from build123d import *

# Parameters (mm, degrees)
SKETCH2_R           = 2
BOSS_EXTRUDE1_DEPTH = 1.7
SKETCH3_W           = 98
SKETCH3_H           = 60
BOSS_EXTRUDE2_DEPTH = 3
SKETCH4_W           = 97
SKETCH4_H           = 40
BOSS_EXTRUDE3_DEPTH = 15
SKETCH5_W           = 6
SKETCH5_H           = 6
BOSS_EXTRUDE4_DEPTH = 3
SKETCH6_R           = 1.75
BOSS_EXTRUDE5_DEPTH = 0.65
SKETCH7_W           = 12.25
SKETCH7_H           = 11.75
BOSS_EXTRUDE6_DEPTH = 4.5
SKETCH8_R           = 6
BOSS_EXTRUDE7_DEPTH = 9.3
SKETCH9_W           = 45
SKETCH9_H           = 22.5
BOSS_EXTRUDE8_DEPTH = 10
SKETCH10_W          = 26.5
SKETCH10_H          = 26.5
BOSS_EXTRUDE9_DEPTH = 3.5
SKETCH11_W          = 76
SKETCH11_H          = 26
CUT_EXTRUDE1_DEPTH  = 0.5


with BuildPart() as part:
    # Sketch2 → Boss-Extrude1 (new body)
    with BuildSketch(Plane.XY):
        Polygon((75, 27.5), (75, -27.5), (-75, -27.5), (-75, 27.5), (-62.25, 27.5), (35.75, 27.5), align=None)
        with Locations((-72.5, -25)):
            Circle(SKETCH2_R, mode=Mode.SUBTRACT)
        with Locations((-72.5, 25)):
            Circle(SKETCH2_R, mode=Mode.SUBTRACT)
        with Locations((72.5, -25)):
            Circle(SKETCH2_R, mode=Mode.SUBTRACT)
        with Locations((72.5, 25)):
            Circle(SKETCH2_R, mode=Mode.SUBTRACT)
    extrude(amount=BOSS_EXTRUDE1_DEPTH)

    # Sketch3 → Boss-Extrude2 (add)
    with BuildSketch(Plane.XY):
        with Locations((-13.25, 6)):
            Rectangle(SKETCH3_W, SKETCH3_H)
    extrude(amount=-BOSS_EXTRUDE2_DEPTH)

    # Sketch4 → Boss-Extrude3 (add)
    with BuildSketch(Plane.XY):
        with Locations((-13.25, 5.5)):
            Rectangle(SKETCH4_W, SKETCH4_H)
    extrude(amount=-BOSS_EXTRUDE3_DEPTH)

    # Sketch5 → Boss-Extrude4 (add)
    with BuildSketch(Plane.XY):
        with Locations((62, 20)):
            Rectangle(SKETCH5_W, SKETCH5_H)
    extrude(amount=-BOSS_EXTRUDE4_DEPTH)

    # Sketch6 → Boss-Extrude5 (add)
    with BuildSketch(Plane(origin=(0, 0, -3), x_dir=(-1, 0, 0), z_dir=(0, 0, -1))):
        with Locations((-62, 20)):
            Circle(SKETCH6_R)
    extrude(amount=BOSS_EXTRUDE5_DEPTH)

    # Sketch7 → Boss-Extrude6 (add)
    with BuildSketch(Plane.XY):
        with Locations((62, 2.5)):
            Rectangle(SKETCH7_W, SKETCH7_H)
    extrude(amount=-BOSS_EXTRUDE6_DEPTH)

    # Sketch8 → Boss-Extrude7 (add)
    with BuildSketch(Plane.XY):
        with Locations((62, -17.5)):
            Circle(SKETCH8_R)
    extrude(amount=-BOSS_EXTRUDE7_DEPTH)

    # Sketch9 → Boss-Extrude8 (add)
    with BuildSketch(Plane.XY.offset(1.7)):
        with Locations((-6.5, 8.75)):
            Rectangle(SKETCH9_W, SKETCH9_H)
    extrude(amount=BOSS_EXTRUDE8_DEPTH)

    # Sketch10 → Boss-Extrude9 (add)
    with BuildSketch(Plane.XY.offset(1.7)):
        with Locations((-61.75, 6.25)):
            Rectangle(SKETCH10_W, SKETCH10_H)
    extrude(amount=BOSS_EXTRUDE9_DEPTH)

    # Sketch11 → Cut-Extrude1 (cut)
    with BuildSketch(Plane(origin=(0, 0, -15), x_dir=(-1, 0, 0), z_dir=(0, 0, -1))):
        with Locations((13.25, 5.5)):
            Rectangle(SKETCH11_W, SKETCH11_H)
    extrude(amount=-CUT_EXTRUDE1_DEPTH, mode=Mode.SUBTRACT)


solid = part.part
The listing builds one solid part. Answer for the finished solid, in the listing's coordinates (mm). A direction names the side the tool comes from. Round coordinates to 2 decimals unless told otherwise and drop trailing zeros. Write each loop counter-clockwise with the first axis right and the second up, starting at its lowest first coordinate (ties: lowest second). Pieces come first, ordered by that corner, then holes. Notation, with made-up numbers: (20.25, 84) - (48.25, 84) arc R22 cw to (48.25, 94) - close; hole circle Ø10 at (-17, -33.75). An arc over 180 degrees is marked (long way). Use a Markdown table: item, result. Add a question column.
1. The part is cut by section A-A (x = 29). Write down the section's boundary in (y, z), and give its area (4 significant figures).
2. Flat-ended cylindrical pins translate along their axes: P1, Ø6.5, axis at x = 72.5, y = -25, coming from the +Z side; P2, Ø4, axis at y = 22.5, z = -8, coming from the +X side; P3, Ø0.8, axis at x = -21.5, z = 0.5, coming from the +Y side; P4, Ø3, axis at x = -72.5, y = -25, coming from the +Z side. Find the tip coordinate at first contact, or state that the pin passes through.
3. The part is cut by section D-D (z = -12.5). Write down the section's boundary in (x, y).
4. For a pull along Y with two mould halves and no side action, classify faces 5 (the face through (56.006, -17.236, -4.585)), 6 (the face through (-14, -24, -1)), 7 (the face through (55.875, 2, -2)), 8 (the face through (-14, 36, -1)) as +Y half, -Y half, draft (parallel to the pull), parting line (faces both ways), or undercut.
5. A tool of negligible diameter and unlimited length cuts with its end or side. For faces 1 (the face through (62, 8.375, -2)), 2 (the face through (-62.25, 6, -1)), 3 (the face through (-48.5, 6, 3)), 4 (the face through (62, 3, -4.5)), from which of +Z, -Z, +X, -X, +Y, -Y can it reach the whole face along a straight path? Write none if from no direction.
6. Consider line 1 (Y direction, x = -72.5, z = 0.75); line 2 (X direction, y = 0, z = -1.5) (3 decimals); line 3 (X direction, y = 0, z = 4.5). Determine where each line is inside the solid, lowest interval first.
7. The part is cut by section B-B (y = 3.5). Write down the section's boundary in (x, z) (3 decimals), and give its area (3 significant figures).
8. The part is cut by section C-C (x = -36.5). Write down the section's boundary in (y, z), and give its area (4 significant figures).
Reported:
| question | item | result |
|---|---|---|
| 1 | outline | (-27.5, 0) - (-24, 0) - (-24, -3) - (-14.5, -3) - (-14.5, -15) - (25.5, -15) - (25.5, -3) - (36, -3) - (36, 0) - (27.5, 0) - (27.5, 1.7) - (-27.5, 1.7) - close |
| 1 | area | 753.5 mm^2 |
| 2 | P1 | z = 1.7 |
| 2 | P2 | x = 35.25 |
| 2 | P3 | y = 27.5 |
| 2 | P4 | through |
| 3 | outline | (-61.75, -14.5) - (35.25, -14.5) - (35.25, 25.5) - (-61.75, 25.5) - close |
| 4 | face 5 | undercut |
| 4 | face 6 | -Y half |
| 4 | face 7 | draft |
| 4 | face 8 | +Y half |
| 5 | face 1 | -Z, +X |
| 5 | face 2 | -Z, -X, +Y, -Y |
| 5 | face 3 | +Z, +Y, -Y |
| 5 | face 4 | -Z, +X, +Y |
| 6 | line 1 | -27.5 to -27, -23 to 23, 27 to 27.5 |
| 6 | line 2 | -62.25 to 35.75, 55.875 to 68.125 |
| 6 | line 3 | -75 to -48.5, -29 to 16 |
| 7 | outline | (-75, 0) - (-62.25, 0) - (-62.25, -3) - (-61.75, -3) - (-61.75, -15) - (-51.25, -15) - (-51.25, -14.5) - (24.75, -14.5) - (24.75, -15) - (35.25, -15) - (35.25, -3) - (35.75, -3) - (35.75, 0) - (55.875, 0) - (55.875, -4.5) - (68.125, -4.5) - (68.125, 0) - (75, 0) - (75, 1.7) - (16, 1.7) - (16, 11.7) - (-29, 11.7) - (-29, 1.7) - (-48.5, 1.7) - (-48.5, 5.2) - (-75, 5.2) - close |
| 7 | area | 2,270 mm^2 |
| 8 | outline | (-27.5, 0) - (-24, 0) - (-24, -3) - (-14.5, -3) - (-14.5, -15) - (-7.5, -15) - (-7.5, -14.5) - (18.5, -14.5) - (18.5, -15) - (25.5, -15) - (25.5, -3) - (36, -3) - (36, 0) - (27.5, 0) - (27.5, 1.7) - (-27.5, 1.7) - close |
| 8 | area | 740.5 mm^2 |
